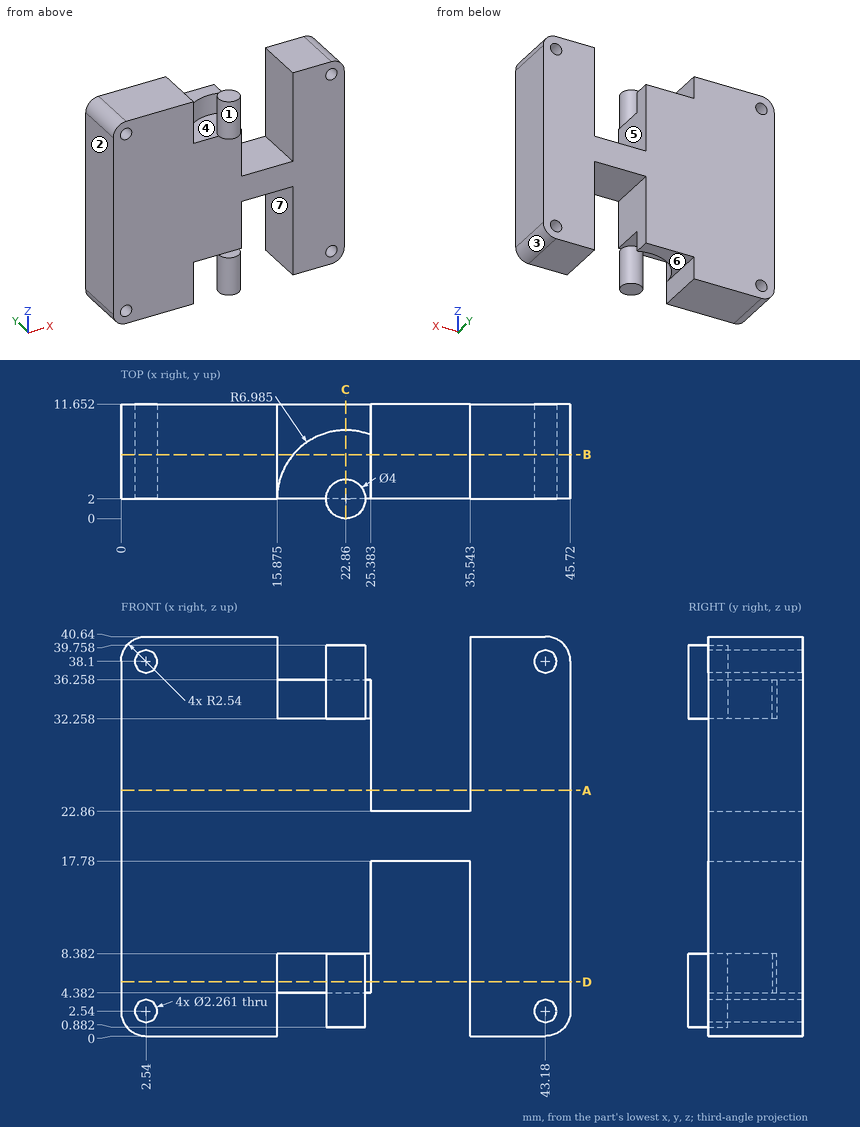
Study the drawing (mm; zero at the part's minimum x, y, z) and answer. A direction names the side the tool comes from. Give positions to 0.01 mm unless a question says otherwise; leave off trailing zeros. Loops run counter-clockwise (first coordinate to the right, second up) from the corner with the lowest first, then second, coordinate; pieces in that order, holes last. Notation, with made-up numbers: (50, 28) -> (54, 28) arc R19 ccw to (54, 32) -> close; hole circle Ø8 at (59.25, 2.5). An arc over 180 degrees is marked (long way). Write item = value, one per line. Start each with the question number.
(1) Find section D-D on z = 5.5. Give the vertices of the cut face in (x, y) (1 decimal).
(2) Find the intervals of material crossed by probe 1 along Z at (x, y) = (43.18, 7); probe 2 along X at (y, z) = (10, 24); probe 3 along X at (y, z) = (4.5, 36.5) (1 decimal), in increasing order. Write a range as from..to.
(3) Find section B-B on y = 6.5. Give the number of separate pieces and of enclosed holes in the cut face, and give its area (3 significant figures).
(4) Given pin 1 Ø2 at (x, y) = (19, 6.5) entering from -Z; pin 2 Ø10 at (x, z) = (12.5, 5.5) entering from -Y; pin 3 Ø2 at (x, y) = (22.5, 1.5) entering from -Z, each flat-ended and moving along its own axis, determine where each tip first touches the part or whether it passes through.
(5) The mould has two halves that part along X. Classify the marked faces 1, 2 and 3: +X half, -X half, draft (parallel to the pull), parting line (faces both ways), or undercut.
(6) Find section A-A on z = 25. Give the vertices of the cut face in (x, y).
(7) Which of the six approach directions +Z, -Z, +X, -X, +Y, -Y give full straight-line access (tool end or side, diameter ignored) to the marked faces 4, 5, 6 and 7?
(8) Find section C-C on x = 22.86. Give the vertices of the cut face in (y, z) (1 decimal).
From the geometry:
q1.outline = (0, 2) -> (15.9, 2) arc R7 cw to (25.4, 8.5) -> (25.4, 11.7) -> (0, 11.7) -> close; circle Ø4 at (22.9, 2); (35.5, 2) -> (45.7, 2) -> (45.7, 11.7) -> (35.5, 11.7) -> close
q2.probe_1 = 0..1.41, 3.67..36.97, 39.23..40.64
q2.probe_2 = 0..25.38, 35.54..45.72
q2.probe_3 = 0..15.9, 35.5..45.7
q3.separate_pieces = 1
q3.enclosed_holes = 4
q3.area = 1,330 mm^2
q4.pin_1 = 8.38
q4.pin_2 = 2
q4.pin_3 = 0.88
q5.face_1 = undercut
q5.face_2 = -X half
q5.face_3 = +X half
q6.outline = (0, 2) -> (25.38, 2) -> (25.38, 11.65) -> (0, 11.65) -> close; (35.54, 2) -> (45.72, 2) -> (45.72, 11.65) -> (35.54, 11.65) -> close
q7.face_4 = +Z
q7.face_5 = +Z, +Y, -Y
q7.face_6 = -Z, +Y
q7.face_7 = -Z, +Y, -Y
q8.outline = (0, 0.9) -> (4, 0.9) -> (4, 8.4) -> (9, 8.4) -> (9, 4.4) -> (11.7, 4.4) -> (11.7, 36.3) -> (9, 36.3) -> (9, 32.3) -> (4, 32.3) -> (4, 39.8) -> (0, 39.8) -> (0, 32.3) -> (2, 32.3) -> (2, 8.4) -> (0, 8.4) -> close
